The listing builds one solid part. Answer for the finished solid, in the listing's coordinates (mm). Round coordinates to 2 decimals unless told otherwise and drop trailing zeros. Loops run counter-clockwise (first coordinate to the right, second up) from the corner with the lowest first, then second, coordinate; pieces in that order, holes last. Notation, with made-up numbers: M -25.5,-40 L 28.5,-40 A20 cw 28.5,-35 Z; hole C 4,55 d4. An arc over 180 degrees is marked long. Answer as a JSON object with one key per item and string values.
```python
from build123d import *

# Parameters (mm, degrees)
SALIENTE_EXTRUIR1_DEPTH = 205
CORTAR_EXTRUIR1_REACH   = 211.458
CROQUIS2_R              = 3
CHAFL_N1_SIZE           = 0.5


with BuildPart() as part:
    # Croquis1 → Saliente-Extruir1 (new, symmetric)
    with BuildSketch(Plane.XY):
        with BuildLine():
            Line((-8.121192263, 10), (-3.67559519, 17.7))
            ThreePointArc((-3.67559519, 17.7), (0, 37), (3.67559519, 17.7))
            Line((3.67559519, 17.7), (8.121192263, 10))
            Line((8.121192263, 10), (9.5, 10))
            Line((9.5, 10), (9.5, 5))
            Line((9.5, 5), (21.88, 5))
            Line((21.88, 5), (21.88, 0))
            Line((21.88, 0), (-21.88, 0))
            Line((-21.88, 0), (-21.88, 5))
            Line((-21.88, 5), (-9.5, 5))
            Line((-9.5, 5), (-9.5, 10))
            Line((-9.5, 10), (-8.121192263, 10))
        make_face()
    extrude(amount=SALIENTE_EXTRUIR1_DEPTH, both=True)

    # Croquis2 → Cortar-Extruir1 (cut, up to next)
    with BuildSketch(Plane.XZ, mode=Mode.PRIVATE) as cortar_extruir1_sk1:
        with Locations(Location((15, 150, 0), (0, 0, 270))):
            Circle(CROQUIS2_R)
    cortar_extruir1_tool1 = extrude(cortar_extruir1_sk1.sketch, amount=-CORTAR_EXTRUIR1_REACH, mode=Mode.PRIVATE) & part.part
    # Croquis2 → Cortar-Extruir1 (cut, up to next)
    with BuildSketch(Plane.XZ, mode=Mode.PRIVATE) as cortar_extruir1_sk2:
        with Locations(Location((-15, 150, 0), (0, 0, 270))):
            Circle(CROQUIS2_R)
    cortar_extruir1_tool2 = extrude(cortar_extruir1_sk2.sketch, amount=-CORTAR_EXTRUIR1_REACH, mode=Mode.PRIVATE) & part.part
    # Croquis2 → Cortar-Extruir1 (cut, up to next)
    with BuildSketch(Plane.XZ, mode=Mode.PRIVATE) as cortar_extruir1_sk3:
        with Locations(Location((-15, 0, 0), (0, 0, 270))):
            Circle(CROQUIS2_R)
    cortar_extruir1_tool3 = extrude(cortar_extruir1_sk3.sketch, amount=-CORTAR_EXTRUIR1_REACH, mode=Mode.PRIVATE) & part.part
    # Croquis2 → Cortar-Extruir1 (cut, up to next)
    with BuildSketch(Plane.XZ, mode=Mode.PRIVATE) as cortar_extruir1_sk4:
        with Locations(Location((15, 0, 0), (0, 0, 270))):
            Circle(CROQUIS2_R)
    cortar_extruir1_tool4 = extrude(cortar_extruir1_sk4.sketch, amount=-CORTAR_EXTRUIR1_REACH, mode=Mode.PRIVATE) & part.part
    # Croquis2 → Cortar-Extruir1 (cut, up to next)
    with BuildSketch(Plane.XZ, mode=Mode.PRIVATE) as cortar_extruir1_sk5:
        with Locations(Location((15, -150, 0), (0, 0, 270))):
            Circle(CROQUIS2_R)
    cortar_extruir1_tool5 = extrude(cortar_extruir1_sk5.sketch, amount=-CORTAR_EXTRUIR1_REACH, mode=Mode.PRIVATE) & part.part
    # Croquis2 → Cortar-Extruir1 (cut, up to next)
    with BuildSketch(Plane.XZ, mode=Mode.PRIVATE) as cortar_extruir1_sk6:
        with Locations(Location((-15, -150, 0), (0, 0, 270))):
            Circle(CROQUIS2_R)
    cortar_extruir1_tool6 = extrude(cortar_extruir1_sk6.sketch, amount=-CORTAR_EXTRUIR1_REACH, mode=Mode.PRIVATE) & part.part
    add(cortar_extruir1_tool1.solids().sort_by_distance((15, 0, 150))[0], mode=Mode.SUBTRACT)
    add(cortar_extruir1_tool2.solids().sort_by_distance((-15, 0, 150))[0], mode=Mode.SUBTRACT)
    add(cortar_extruir1_tool3.solids().sort_by_distance((-15, 0, 0))[0], mode=Mode.SUBTRACT)
    add(cortar_extruir1_tool4.solids().sort_by_distance((15, 0, 0))[0], mode=Mode.SUBTRACT)
    add(cortar_extruir1_tool5.solids().sort_by_distance((15, 0, -150))[0], mode=Mode.SUBTRACT)
    add(cortar_extruir1_tool6.solids().sort_by_distance((-15, 0, -150))[0], mode=Mode.SUBTRACT)

    # Chaflán1
    chafl_n1_edges = [part.edges().sort_by_distance(p)[0] for p in [
        (-15, 5, 153),
        (-15, 5, 3),
        (15, 5, 3),
        (15, 5, -147),
        (-15, 5, -147),
        (15, 5, 153),
    ]]
    chamfer(chafl_n1_edges, length=CHAFL_N1_SIZE)


solid = part.part
```
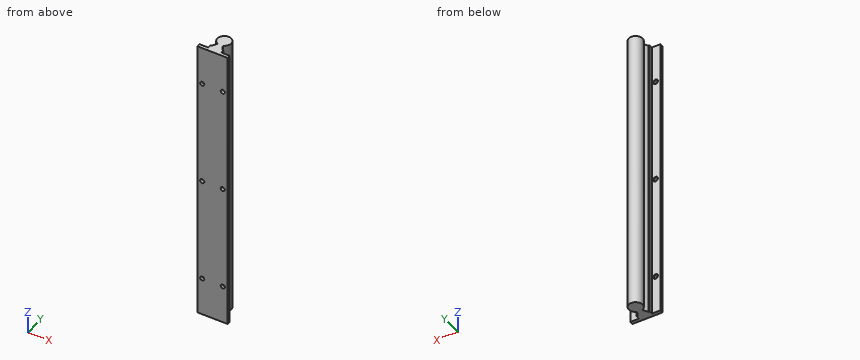
Item 1: Straight lines are drawn through the part: line 1 (X direction, y = 1.8, z = -150); line 2 (Y direction, x = 1, z = 15.5); line 3 (Y direction, x = -12, z = 94). For each, find the intervals that lie inside material, in ascending order.
Values follow:
{"line 1": "-21.88 to -18, -12 to 12, 18 to 21.88", "line 2": "0 to 36.95", "line 3": "0 to 5"}
Item 2: The part is cut by section A-A (z = -159). Give the vertices of the cut face in (x, y), then the cut area to 3 significant figures.
Values follow:
{"outline": "M -21.88,0 L 21.88,0 L 21.88,5 L 9.5,5 L 9.5,10 L 8.12,10 L 3.68,17.7 A10 ccw long -3.68,17.7 L -8.12,10 L -9.5,10 L -9.5,5 L -21.88,5 Z", "area": "715 mm^2"}
Item 3: The part is cut by section B-B (y = 27). Give the vertices of the cut face in (x, z).
Values follow:
{"outline": "M -10,-205 L 10,-205 L 10,205 L -10,205 Z"}
Item 4: Flat-ended cylindrical pins translate along their axes: P1, Ø3, axis at x = 2.5, z = -163, coming from the +Y side; P2, Ø4, axis at y = 25, z = -136, coming from the -X side; P3, Ø10, axis at x = 17.5, z = -48, coming from the +Y side. Find the tip coordinate at first contact, or state that the pin passes through.
Values follow:
{"P1": "y = 36.95", "P2": "x = -10", "P3": "y = 5"}
